from build123d import *

# Parameters (mm, degrees)
F1_DEPTH = 48.350064
F2_R     = 5.08
F4_R     = 19.298697
F5_DEPTH = 25.4


with BuildPart() as f1:
    # F0 (on Top) → F1 (new body)
    with BuildSketch(Plane.XY):
        Polygon((107.200803, -20.653679), (-77.255428, 73.898613), (30.614838, -75.829387), align=None)
    extrude(amount=F1_DEPTH)

    # F2
    f2_edges = [f1.edges().sort_by_distance(p)[0] for p in [
        (-77.255428, 73.898613, 24.175032),
        (68.90782, -48.241533, 48.350064),
        (107.200803, -20.653679, 24.175032),
        (14.972687, 26.622467, 0),
        (14.972687, 26.622467, 48.350064),
        (-23.320295, -0.965387, 0),
        (68.90782, -48.241533, 0),
        (30.614838, -75.829387, 24.175032),
        (-23.320295, -0.965387, 48.350064),
    ]]
    fillet(f2_edges, radius=F2_R)

    # F4 (on face) → F5 (join)
    with BuildSketch(Plane.XY.offset(48.350064)):
        with Locations((31.383455, -22.975024)):
            Circle(F4_R)
    extrude(amount=F5_DEPTH)


solid = f1.part
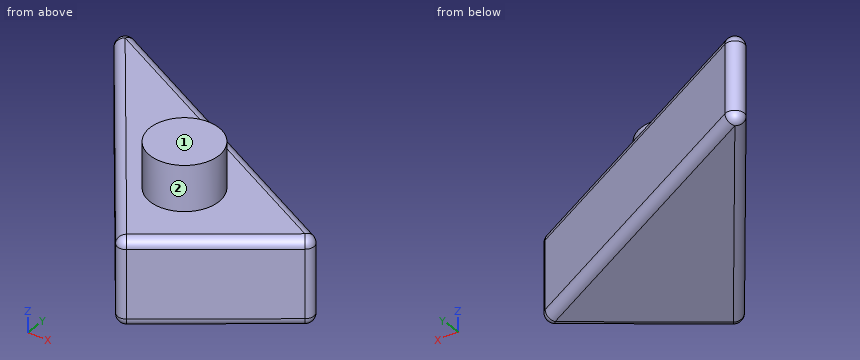
For this review, take the finished solid that the model builds, in its own axes (mm). Face numbers are marked on the shaded views. A direction names the side the tool comes from. Give positions to 0.01 mm unless a question says otherwise; leave off trailing zeros. Order: outer loops, then holes, each group sorted by start corner. A loop starts at its lowest first (then second) coordinate and runs counter-clockwise, first axis right, second up. Notation, with made-up numbers: M 74,59.25 L 108,59.25 A27 cw 108,75.25 Z; hole C 22.5,31.5 d1. An arc over 180 degrees is marked long. Answer in a Markdown table with one row per item. Add a question column.
(1) For the marked faces 1 and 2, list the 3-axis set-ups (+Z, -Z, +X, -X, +Y, -Y) from which the entire face can be reached by the end or side of a thin tool; tool diameter is ignored.
(2) For pin 1 (1 mm diameter, centred on x = 33.5, z = 30.5, fed in from -Y); pin 2 (2 mm diameter, centred on x = 79, y = -31, fed in from +Z); pin 3 (6 mm diameter, centred on x = -43, z = 30, fed in from -Y), all flat-tipped, find the tip position at first contact; note any pin that passes through.
(3) Consider section B-B on z = 61. State the section outline as (x, y) points, and give its area (3 significant figures).
(4) Wall thickness on probe 1 along Z at (x, y) = (60, -27.5); probe 2 along X at (y, z) = (-14, 70.5); probe 3 along Z at (x, y) = (40, 13): over which ranges is each line inside the solid? List them lowest first. Write a range as [from, to].
(5) Consider section A-A on z = 38. State the section outline as (x, y) points.
Evaluation:
| question | item | result |
|---|---|---|
| 1 | face 1 | +Z, +X, -X, +Y, -Y |
| 1 | face 2 | +Z |
| 2 | pin 1 | stops at y = -73.67 |
| 2 | pin 2 | stops at z = 48.35 |
| 2 | pin 3 | stops at y = 22.19 |
| 3 | outline | C 31.38,-22.98 d38.6 |
| 3 | area | 1,170 mm^2 |
| 4 | probe 1 | z = [0, 48.35] |
| 4 | probe 2 | x = [14.3, 48.47] |
| 4 | probe 3 | z = [2.5, 45.85] |
| 5 | outline | M -64.93,56.79 L 27.65,-71.71 A5.08 ccw 34.74,-72.86 L 100.46,-25.51 A5.08 ccw 99.81,-16.87 L -58.49,64.28 A5.08 ccw Z |
